```python
from build123d import *

# Parameters (mm, degrees)
SKETCH1_W               = 32.75
SKETCH1_H               = 190
BOSS_EXTRUDE1_DEPTH     = 3.5
SKETCH3_R               = 1.5
CUT_EXTRUDE1_DEPTH      = 97.46445265
MIRROR2_COPY_1_SKETCH_R = 1.5
MIRROR2_COPY_1_DEPTH    = 97.46445265
SKETCH4_R               = 1.5
CUT_EXTRUDE2_DEPTH      = 97.46445265
MIRROR4_COPY_1_SKETCH_R = 1.5
MIRROR4_COPY_1_DEPTH    = 97.46445265
BOSS_EXTRUDE2_DEPTH     = 3.5
FILLET1_R               = 10
FILLET2_R               = 10
FILLET5_R               = 10
FILLET6_R               = 10
MIRROR14_COPY_1_DEPTH   = 3.5
FILLET7_R               = 10
FILLET8_R               = 10
CUT_EXTRUDE3_DEPTH      = 102.304491633


with BuildPart() as part:
    # Sketch1 → Boss-Extrude1 (new body)
    with BuildSketch(Plane(origin=(0, 0, 0), x_dir=(1, 0, 0), z_dir=(0, 1, 0))):
        Rectangle(SKETCH1_W, SKETCH1_H)
    extrude(amount=BOSS_EXTRUDE1_DEPTH)

    # Sketch3 → Cut-Extrude1 (cut, through all)
    with BuildSketch(Plane(origin=(0, 3.5, 0), x_dir=(1, 0, 0), z_dir=(0, 1, 0))):
        with Locations(Location((-12.375, -46.625, 0), (0, 0, 270))):
            Circle(SKETCH3_R)
        with Locations(Location((-12.375, -78.625, 0), (0, 0, 270))):
            Circle(SKETCH3_R)
        Polygon((-16.375, -95), (-8.5, -95), (-16.375, -80.125), align=None)
    cut_extrude1 = extrude(amount=-CUT_EXTRUDE1_DEPTH, mode=Mode.SUBTRACT)

    # Mirror1: Cut-Extrude1 across plane
    add(cut_extrude1.mirror(Plane(origin=(0, 0, 0), x_dir=(0, 0, 1), z_dir=(1, 0, 0))), mode=Mode.SUBTRACT)

    # Mirror2: Cut-Extrude1 across plane
    add(cut_extrude1.mirror(Plane.XY), mode=Mode.SUBTRACT)

    # Mirror2 copy 1 sketch → Mirror2 copy 1 (cut, through all)
    with BuildSketch(Plane(origin=(0, 3.5, 0), x_dir=(-1, 0, 0), z_dir=(0, 1, 0))):
        with Locations(Location((-12.375, -46.625, 0), (0, 0, 270))):
            Circle(MIRROR2_COPY_1_SKETCH_R)
        with Locations(Location((-12.375, -78.625, 0), (0, 0, 270))):
            Circle(MIRROR2_COPY_1_SKETCH_R)
        Polygon((-16.375, -95), (-8.5, -95), (-16.375, -80.125), align=None)
    extrude(amount=-MIRROR2_COPY_1_DEPTH, mode=Mode.SUBTRACT)

    # Sketch4 → Cut-Extrude2 (cut, through all)
    with BuildSketch(Plane(origin=(0, 3.5, 0), x_dir=(1, 0, 0), z_dir=(0, 1, 0))):
        with Locations(Location((5.375, -75.065, 0), (0, 0, 270))):
            Circle(SKETCH4_R)
    cut_extrude2 = extrude(amount=-CUT_EXTRUDE2_DEPTH, mode=Mode.SUBTRACT)

    # Mirror3: Cut-Extrude2 across plane
    add(cut_extrude2.mirror(Plane(origin=(0, 0, 0), x_dir=(0, 0, 1), z_dir=(1, 0, 0))), mode=Mode.SUBTRACT)

    # Mirror4: Cut-Extrude2 across plane
    add(cut_extrude2.mirror(Plane.XY), mode=Mode.SUBTRACT)

    # Mirror4 copy 1 sketch → Mirror4 copy 1 (cut, through all)
    with BuildSketch(Plane(origin=(0, 3.5, 0), x_dir=(-1, 0, 0), z_dir=(0, 1, 0))):
        with Locations(Location((5.375, -75.065, 0), (0, 0, 270))):
            Circle(MIRROR4_COPY_1_SKETCH_R)
    extrude(amount=-MIRROR4_COPY_1_DEPTH, mode=Mode.SUBTRACT)

    # Sketch5 → Boss-Extrude2 (add)
    with BuildSketch(Plane.XZ):
        with BuildLine():
            Line((17.375, 29.995), (16.375, 29.995))
            Line((16.375, 29.995), (16.375, 24.995))
            Line((16.375, 24.995), (16.375, 19.995))
            Line((16.375, 19.995), (30.005, 19.995))
            ThreePointArc((30.005, 19.995), (35.005, 24.995), (30.005, 29.995))
            Line((30.005, 29.995), (17.375, 29.995))
        make_face()
        with BuildLine():
            ThreePointArc((31.005, 24.995), (30.005, 23.995), (29.005, 24.995))
            ThreePointArc((29.005, 24.995), (30.005, 25.995), (31.005, 24.995))
        make_face(mode=Mode.SUBTRACT)
    boss_extrude2 = extrude(amount=-BOSS_EXTRUDE2_DEPTH)

    # Fillet1
    fillet1_edges = [part.edges().sort_by_distance(p)[0] for p in [
        (16.375, 1.75, 29.995),
    ]]
    fillet(fillet1_edges, radius=FILLET1_R)

    # Fillet2
    fillet2_edges = [part.edges().sort_by_distance(p)[0] for p in [
        (16.375, 1.75, 19.995),
    ]]
    fillet(fillet2_edges, radius=FILLET2_R)

    # Mirror13: Boss-Extrude2 across plane
    add(boss_extrude2.mirror(Plane(origin=(0, 0, 0), x_dir=(0, 0, 1), z_dir=(1, 0, 0))))

    # Fillet5
    fillet5_edges = [part.edges().sort_by_distance(p)[0] for p in [
        (-16.375, 1.75, 29.995),
    ]]
    fillet(fillet5_edges, radius=FILLET5_R)

    # Fillet6
    fillet6_edges = [part.edges().sort_by_distance(p)[0] for p in [
        (-16.375, 1.75, 19.995),
    ]]
    fillet(fillet6_edges, radius=FILLET6_R)

    # Mirror14: Boss-Extrude2 across plane
    add(boss_extrude2.mirror(Plane.XY))

    # Mirror14 copy 1 sketch → Mirror14 copy 1 (add)
    with BuildSketch(Plane(origin=(0, 0, 0), x_dir=(-1, 0, 0), z_dir=(0, -1, 0))):
        with BuildLine():
            Line((17.375, 29.995), (16.375, 29.995))
            Line((16.375, 29.995), (16.375, 24.995))
            Line((16.375, 24.995), (16.375, 19.995))
            Line((16.375, 19.995), (30.005, 19.995))
            ThreePointArc((30.005, 19.995), (35.005, 24.995), (30.005, 29.995))
            Line((30.005, 29.995), (17.375, 29.995))
        make_face()
        with BuildLine():
            ThreePointArc((31.005, 24.995), (30.005, 23.995), (29.005, 24.995))
            ThreePointArc((29.005, 24.995), (30.005, 25.995), (31.005, 24.995))
        make_face(mode=Mode.SUBTRACT)
    extrude(amount=-MIRROR14_COPY_1_DEPTH)

    # Fillet7
    fillet7_edges = [part.edges().sort_by_distance(p)[0] for p in [
        (-16.375, 1.75, -29.995),
    ]]
    fillet(fillet7_edges, radius=FILLET7_R)

    # Fillet8
    fillet8_edges = [part.edges().sort_by_distance(p)[0] for p in [
        (-16.375, 1.75, -19.995),
    ]]
    fillet(fillet8_edges, radius=FILLET8_R)

    # Sketch6 → Cut-Extrude3 (cut, through all)
    with BuildSketch(Plane(origin=(0, 3.5, 0), x_dir=(1, 0, 0), z_dir=(0, 1, 0))):
        Polygon((16.375, 5), (16.375, 44.924773713), (47.716486095, 44.924773713), (47.716486095, -55.8941685), (16.375, -55.8941685), align=None)
    extrude(amount=-CUT_EXTRUDE3_DEPTH, mode=Mode.SUBTRACT)


solid = part.part
```
The model under review builds one solid part; all positions refer to its coordinate system, in mm. A direction names the side the tool comes from. Round coordinates to 2 decimals unless told otherwise and drop trailing zeros. Loops run counter-clockwise (first coordinate to the right, second up) from the corner with the lowest first, then second, coordinate; pieces in that order, holes last.
Item 1: Mouldability with a two-part tool opening along Z and no side actions: class faces 3 (the face through (-19.23, 1.77, 33)), 4 (the face through (5.441, 1.774, 73.566)), 5 (the face through (-4, 3.5, -1)), 6 (the face through (-28, 2, -29.995)) as released by +Z, released by -Z, zero draft, split by the parting line, or undercut.
Determined:
face 3: released by +Z
face 4: undercut
face 5: zero draft
face 6: released by -Z
Item 2: Take a section at A-A (x = -24). Write out the cut boundary in (y, z), then the cut area to 3 significant figures.
Determined:
outline: (0, -30.28) - (3.5, -30.28) - (3.5, -19.71) - (0, -19.71) - close; (0, 19.71) - (3.5, 19.71) - (3.5, 30.28) - (0, 30.28) - close
area: 74.0 mm2
Item 3: Clearance check with flat-ended pins moving along their axes: pin 1 Ø4 at (x, z) = (12.375, 46.625) entering from +Y; pin 2 Ø1.8 at (y, z) = (1.5, 4) entering from -X (3 decimals); pin 3 Ø2 at (x, y) = (10, 2) entering from +Z; pin 4 Ø1 at (x, y) = (-27.5, 2.5) entering from -Z (3 decimals). State where each tip first meets the part, or that it passes through.
Determined:
pin 1: stops at y = 3.5
pin 2: stops at x = -16.375
pin 3: stops at z = 94.06
pin 4: stops at z = -29.995
Item 4: For line 1 (Z direction, x = 12, y = 1.7); line 2 (X direction, y = 2.75, z = -43.5) (3 decimals); line 3 (X direction, y = 0.45, z = -25) (3 decimals), list the stretches that pass through material, from the lowest coordinate up.
Determined:
line 1: z = -88.39 to -80.08, -77.17 to -48.08, -45.17 to 45.17, 48.08 to 77.17, 80.08 to 88.39
line 2: x = -16.375 to 16.375
line 3: x = -35.005 to -31.005, -29.005 to 16.375
Item 5: Take a section at C-C (z = -69.5). Write out the cut boundary in (x, y) (3 decimals), then the cut area to 3 significant figures.
Determined:
outline: (-16.375, 0) - (16.375, 0) - (16.375, 3.5) - (-16.375, 3.5) - close
area: 115 mm2
Item 6: Take a section at D-D (z = -14.5). Write out the cut boundary in (x, y) (3 decimals).
Determined:
outline: (-17.447, 0) - (16.375, 0) - (16.375, 3.5) - (-17.447, 3.5) - close
Item 7: For faces 1 (the face through (-16.375, 2, 0)), 2 (the face through (-11.924, 1.774, -80.056)), list the 3-axis set-ups (+Z, -Z, +X, -X, +Y, -Y) from which the entire face can be reached by the end or side of a thin tool; tool diameter is ignored.
Determined:
face 1: -X, +Y, -Y
face 2: +Y, -Y
Item 8: Take a section at B-B (y = 0.9). Give the number of separate pieces and of enclosed holes in the cut face, then the cut area to 3 significant figures.
Determined:
separate pieces: 1
enclosed holes: 14
area: 6,330 mm2
